Can you work these out from the model? Positions are in its coordinate system, mm. Coordinates: 2 decimals unless noted, no trailing zeros. Order: outer loops, then holes, each group sorted by start corner. A loop starts at its lowest first (then second) coordinate and runs counter-clockwise, first axis right, second up. Notation, with made-up numbers: (-18, 88) - (14, 88) arc R11 cw to (14, 102) - close; hole circle Ø2 at (28, 73). An arc over 180 degrees is marked (long way). Use a Markdown table: item, result. Add a question column.
(1) If I drill on L1, parallel to Y at x = -10, z = 2; L2, parallel to X at y = -3.75, z = 1.5; L3, parallel to X at y = -4, z = 0.75, over which ranges is the centre line in solid material (lowest first)? Write a range as [from, to].
(2) I want a section at A-A (x = -17.5). List the corners of the cut face in (y, z) for me, and give its area (3 significant figures).
(3) I want a section at B-B (z = 2.65). List the corners of the cut face in (x, y) for me, and give its area (3 significant figures).
(4) I want a section at C-C (y = 0). List the corners of the cut face in (x, z) for me, and give its area (3 significant figures).
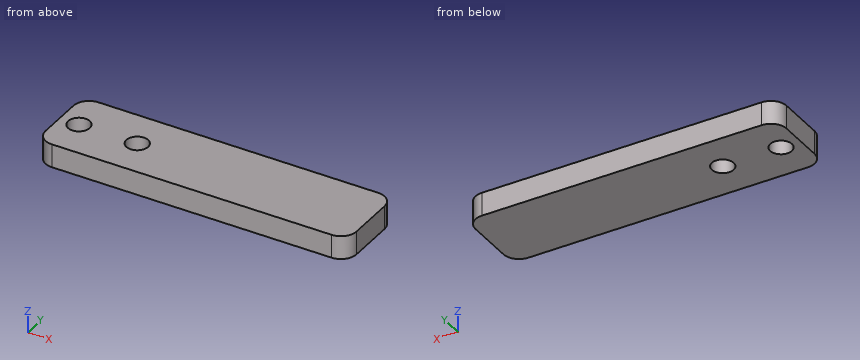
```python
from build123d import *

# Parameters (mm, degrees)
ESQUISSE1_W        = 40
ESQUISSE1_H        = 10
ESQUISSE1_R        = 1.4
BOSS_EXTRU_1_DEPTH = 3
CONG_1_R           = 2


with BuildPart() as part:
    # Esquisse1 → Boss.-Extru.1 (new body)
    with BuildSketch(Plane.XY):
        Rectangle(ESQUISSE1_W, ESQUISSE1_H)
        with Locations((-10, 0)):
            Circle(ESQUISSE1_R, mode=Mode.SUBTRACT)
        with Locations((-17.5, 0)):
            Circle(ESQUISSE1_R, mode=Mode.SUBTRACT)
    extrude(amount=BOSS_EXTRU_1_DEPTH)

    # Congé1
    cong_1_edges = [part.edges().sort_by_distance(p)[0] for p in [
        (20, -5, 1.5),
        (-20, -5, 1.5),
        (-20, 5, 1.5),
        (20, 5, 1.5),
    ]]
    fillet(cong_1_edges, radius=CONG_1_R)


solid = part.part
```
Answers follow:
| question | item | result |
|---|---|---|
| 1 | L1 | y = [-5, -1.4], [1.4, 5] |
| 1 | L2 | x = [-19.85, 19.85] |
| 1 | L3 | x = [-19.73, 19.73] |
| 2 | outline | (-5, 0) - (-1.4, 0) - (-1.4, 3) - (-5, 3) - close; (1.4, 0) - (5, 0) - (5, 3) - (1.4, 3) - close |
| 2 | area | 21.6 mm² |
| 3 | outline | (-20, -3) arc R2 ccw to (-18, -5) - (18, -5) arc R2 ccw to (20, -3) - (20, 3) arc R2 ccw to (18, 5) - (-18, 5) arc R2 ccw to (-20, 3) - close; hole circle Ø2.8 at (-17.5, 0); hole circle Ø2.8 at (-10, 0) |
| 3 | area | 384 mm² |
| 4 | outline | (-20, 0) - (-18.9, 0) - (-18.9, 3) - (-20, 3) - close; (-16.1, 0) - (-11.4, 0) - (-11.4, 3) - (-16.1, 3) - close; (-8.6, 0) - (20, 0) - (20, 3) - (-8.6, 3) - close |
| 4 | area | 103 mm² |
